from build123d import *

# Parameters (mm, degrees)
CIRPATTERN1_COUNT = 4
CIRPATTERN2_COUNT = 4


with BuildPart() as part:
    # Sketch1 → Revolve2 (revolve)
    with BuildSketch(Plane.XY, mode=Mode.PRIVATE) as revolve2_sk:
        Polygon((19.839067821, 36.426477833), (24.767495434, 36.426477833), (24.767495434, 14.248399015), (51.887938783, 14.248399015), (51.887938783, -7.976600985), (14.87066517, -7.976600985), (14.87066517, 26.379705263), (19.839067821, 26.379705263), align=None)
    revolve(revolve2_sk.sketch.rotate(Axis((0, 36.426477833, 0), (0, -1, 0)), 90), axis=Axis((0, 36.426477833, 0), (0, -1, 0)))

    # Sketch4 → 1/4-20 Tapped Hole2 (revolve, cut)
    with BuildSketch(Plane(origin=(42.533479959, 14.248399015, 7.295039057), x_dir=(0, 0, 1), z_dir=(1, 0, 0))):
        Polygon((0, 0), (0, 18.043816902), (2.5527, 16.51), (2.5527, 12.7), (3.175, 12.7), (3.175, 0), align=None)
    f_1_4_20_tapped_hole2 = revolve(axis=Axis((42.533479959, 20.598399015, 7.295039057), (0, -1, 0)), mode=Mode.SUBTRACT)

    # CirPattern1: 1/4-20 Tapped Hole2 ×4 about axis
    cirpattern1_axis = Axis((0, 0, 0), (0, 1, 0))
    for i in range(1, CIRPATTERN1_COUNT):
        add(f_1_4_20_tapped_hole2.rotate(cirpattern1_axis, i * 360 / CIRPATTERN1_COUNT), mode=Mode.SUBTRACT)

    # Sketch7 → CBORE for #10 Binding Head Machine Screw1 (revolve, cut)
    with BuildSketch(Plane(origin=(35.234083692, 14.248399015, -24.91734052), x_dir=(0, 0, 1), z_dir=(1, 0, 0))):
        Polygon((0, 0), (0, 22.225), (2.5527, 22.225), (2.5527, 3.1242), (5.55625, 3.1242), (5.55625, 0.635), (6.19125, 0), align=None)
    cbore_for_10_binding_head_machine_screw = revolve(axis=Axis((35.234083692, 20.598399015, -24.91734052), (0, -1, 0)), mode=Mode.SUBTRACT)

    # CirPattern2: CBORE for #10 Binding Head Machine Screw1 ×4 about axis
    cirpattern2_axis = Axis((0, 0, 0), (0, 1, 0))
    for i in range(1, CIRPATTERN2_COUNT):
        add(cbore_for_10_binding_head_machine_screw.rotate(cirpattern2_axis, i * 360 / CIRPATTERN2_COUNT), mode=Mode.SUBTRACT)


solid = part.part
Geometry: final body of the model. Coordinates: model frame, mm. A direction names the side the tool comes from. Round coordinates to 2 decimals unless told otherwise and drop trailing zeros. Loops run counter-clockwise (first coordinate to the right, second up) from the corner with the lowest first, then second, coordinate; pieces in that order, holes last. Notation, with made-up numbers: (56, 82) - (77, 82) arc R5 ccw to (77, 89) - close; hole circle Ø6 at (72.25, 46.5). An arc over 180 degrees is marked (long way). Write each question's results on one line, items separated by ' | '. Start each with the question number.
1) Cut plane A-A on z = 0. Return loops of the section in (x, y), then the cut area to 3 significant figures.
2) Mould query, pull axis Z, two halves, no side actions, for faces 1 (the face through (-15.59, 2.98, 49.49)), 2 (the face through (23.55, 1.71, 33.08)), 3 (the face through (-20, 36.426, 0)). Classes: released by +Z, released by -Z, zero draft, split by the parting line, or undercut.
3) Access query for faces 4 (the face through (22.35, 12.39, 40.16)), 5 (the face through (13.193, 9.442, 6.862)). Directions: +Z, -Z, +X, -X, +Y, -Y. A direction counts if a zero-diameter tool reaches every point of the face in a straight line with its end or side. Return the directions, or none.
4) Cut plane B-B on x = 0. Return loops of the section in (y, z), then the cut area to 3 significant figures.
5) Line query: probe 1 along X at (y, z) = (32, 0); probe 2 along Y at (x, z) = (-9, -31.5); probe 3 along X at (y, z) = (17, 0). Output: solid intervals per line, ascending. Write a range as [from, to].
6) First-contact query: P1, Ø1, axis at x = -35, z = 6, coming from the +Y side; P2, Ø3, axis at x = -26, y = 5.5, coming from the -Z side; P3, Ø20, axis at x = 9.5, z = 3, coming from the +Y side; P4, Ø9, axis at x = 23.5, z = 35, coming from the +Y side. Flat tips, straight axial feed; report the tip coordinate or a pass-through.
7) Cut plane C-C on y = 25. Return loops of the section in (x, z) (1 decimal).
Verdict:
1) outline: (-51.89, -7.98) - (-14.87, -7.98) - (-14.87, 26.38) - (-19.84, 26.38) - (-19.84, 36.43) - (-24.77, 36.43) - (-24.77, 14.25) - (-51.89, 14.25) - close; (14.87, -7.98) - (51.89, -7.98) - (51.89, 14.25) - (24.77, 14.25) - (24.77, 36.43) - (19.84, 36.43) - (19.84, 26.38) - (14.87, 26.38) - close | area: 1,980 mm2
2) face 1: split by the parting line | face 2: undercut | face 3: zero draft
3) face 4: +Y | face 5: +Y, -Y
4) outline: (-7.98, -51.89) - (14.25, -51.89) - (14.25, -24.77) - (36.43, -24.77) - (36.43, -19.84) - (26.38, -19.84) - (26.38, -14.87) - (-7.98, -14.87) - close; (-7.98, 14.87) - (26.38, 14.87) - (26.38, 19.84) - (36.43, 19.84) - (36.43, 24.77) - (14.25, 24.77) - (14.25, 51.89) - (-7.98, 51.89) - close | area: 1,980 mm2
5) probe 1: x = [-24.77, -19.84], [19.84, 24.77] | probe 2: y = [-7.98, 14.25] | probe 3: x = [-24.77, -14.87], [14.87, 24.77]
6) P1: stops at y = 14.25 | P2: stops at z = -45.74 | P3: stops at y = 36.43 | P4: stops at y = 13.99
7) outline: circle Ø49.5 at (0, 0); hole circle Ø29.7 at (0, 0)
